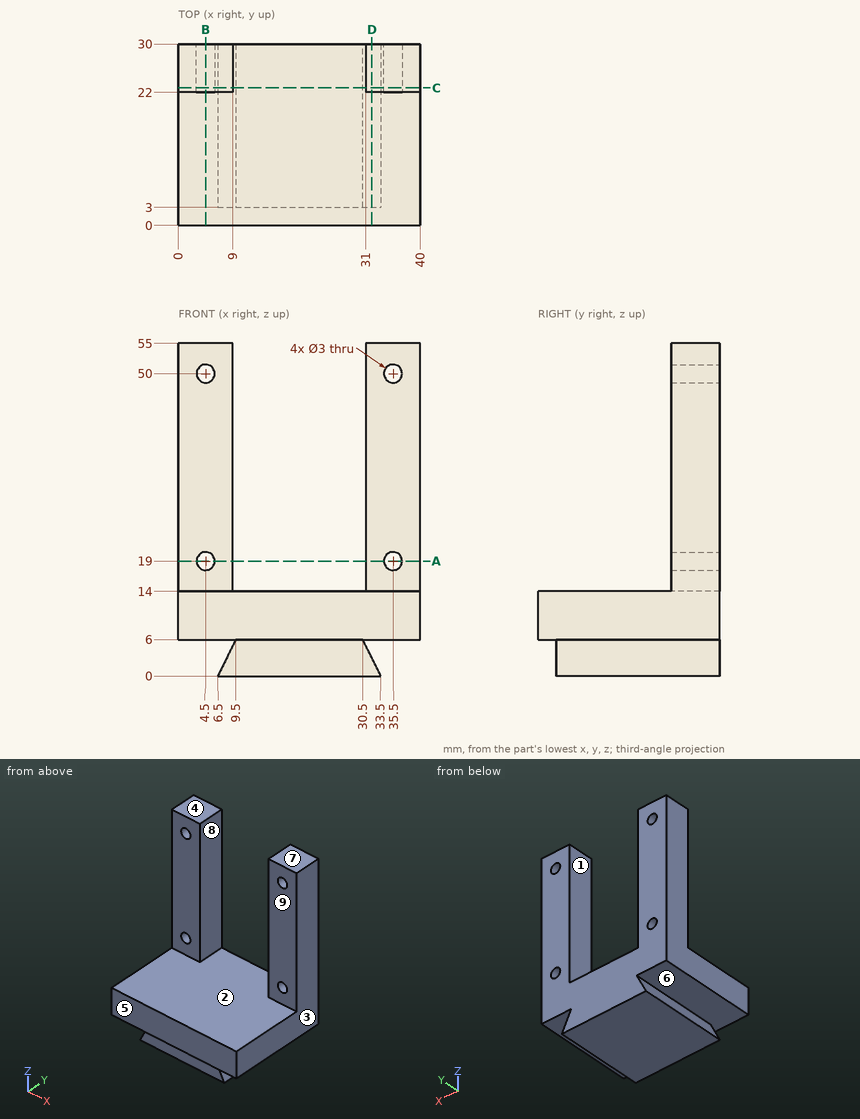
Can you work these out from the drawing? Everything is in mm from the part's minimum corner. A direction names the side the tool comes from. Coordinates: 2 decimals unless noted, no trailing zeros. Loops run counter-clockwise (first coordinate to the right, second up) from the corner with the lowest first, then second, coordinate; pieces in that order, holes last.
1. Imagine slicing it at A-A, the plane z = 19. Please give me the cut outline in (x, y).
2. Imagine slicing it at D-D, the plane x = 32. Please give me the cut outline in (y, z), and give its area (3 significant figures).
3. If we mould it in two halves opening along X, with no side actions, what happens to the marked faces 1, 2, 3 and 4? For each: pulls with the +X half, pulls with the -X half, needs draft (parallel to the pull), parting line crosses it, or undercut.
4. I need wall thicknesses on L1, parallel to Z at x = 4.5, y = 25.5; L2, parallel to X at y = 28.25, z = 47; L3, parallel to X at y = 28.25, z = 18. Which ranges of each line are inside material? Lowest first, please.
5. Imagine slicing it at C-C, the plane y = 22.75. Please give me the cut outline in (x, z).
6. For P1, Ø1, axis at x = 19.5, y = 26.5, coming from the +Z side; P2, Ø7, axis at x = 36.5, z = 26.5, coming from the -Y side; P3, Ø5, axis at x = 18, z = 3, coming from the -Y side, each with a flat end and sliding along its axis, tell me the tip position at first contact or that it passes through.
7. Imagine slicing it at B-B, the plane x = 4.5. Please give me the cut outline in (y, z).
8. For the marked faces 5, 6, 7, 8 and 9, which set-ups out of +Z, -Z, +X, -X, +Y, -Y let a thin tool reach every point of the face, with its end or its side?
Taken from the geometry:
1. outline: (0, 22) - (3, 22) - (3, 30) - (0, 30) - close; (6, 22) - (9, 22) - (9, 30) - (6, 30) - close; (31, 22) - (34, 22) - (34, 30) - (31, 30) - close; (37, 22) - (40, 22) - (40, 30) - (37, 30) - close
2. outline: (0, 6) - (30, 6) - (30, 55) - (22, 55) - (22, 14) - (0, 14) - close; (3, 0) - (30, 0) - (30, 3) - (3, 3) - close
2. area: 649 mm2
3. face 1: undercut
3. face 2: undercut
3. face 3: pulls with the +X half
3. face 4: needs draft
4. L1: z = 6 to 17.5, 20.5 to 48.5, 51.5 to 55
4. L2: x = 0 to 9, 31 to 40
4. L3: x = 0 to 3.38, 5.62 to 9, 31 to 34.38, 36.62 to 40
5. outline: (0, 6) - (9.5, 6) - (6.5, 0) - (33.5, 0) - (30.5, 6) - (40, 6) - (40, 55) - (31, 55) - (31, 14) - (9, 14) - (9, 55) - (0, 55) - close; hole circle Ø3 at (4.5, 19); hole circle Ø3 at (4.5, 50); hole circle Ø3 at (35.5, 19); hole circle Ø3 at (35.5, 50)
6. P1: stops at z = 14
6. P2: stops at y = 22
6. P3: stops at y = 3
7. outline: (0, 6) - (30, 6) - (30, 17.5) - (22, 17.5) - (22, 14) - (0, 14) - close; (22, 20.5) - (30, 20.5) - (30, 48.5) - (22, 48.5) - close; (22, 51.5) - (30, 51.5) - (30, 55) - (22, 55) - close
8. face 5: +Z, -Z, +X, -X, -Y
8. face 6: -Y
8. face 7: +Z, +X, -X, +Y, -Y
8. face 8: +Z, +Y, -Y
8. face 9: +Z, +X, -X, -Y
